```python
from build123d import *

# Parameters (mm, degrees)
EXTRUDE_1_DEPTH          = 60
CUT_EXTRUDE_1_DEPTH      = 40
CUT_EXTRUDE_1_DEPTH_BACK = 29
SKETCH_4_R               = 15.5
SKETCH_5_W               = 5
SKETCH_5_H               = 30
CUT_EXTRUDE_2_DEPTH      = 83.900874001
CUT_EXTRUDE_START        = 25
SKETCH_6_W               = 60
SKETCH_6_H               = 56
CUT_EXTRUDE_3_DEPTH      = 10
CUT_EXTRUDE_START_2      = -15
SKETCH_7_W               = 60
SKETCH_7_H               = 56
CUT_EXTRUDE_4_DEPTH      = 10


with BuildPart() as part:
    # 스케치3 → 보스-돌출1 (new body)
    with BuildSketch(Plane(origin=(0, 0, 0), x_dir=(0, 0, -1), z_dir=(1, 0, 0))):
        Polygon((-25, -51.454396413), (25, -51.454396413), (15, 4.545603587), (-15, 4.545603587), align=None)
    extrude(amount=EXTRUDE_1_DEPTH)

    # 스케치4 → 컷-돌출1 (cut, two sides: drawn at the far end of the back side and taken through both)
    with BuildSketch(Plane.XY.offset(-CUT_EXTRUDE_1_DEPTH_BACK)):
        with Locations(Location((30, -14.954396413, 0), (0, 0, 90))):
            Circle(SKETCH_4_R)
    extrude(amount=CUT_EXTRUDE_1_DEPTH + CUT_EXTRUDE_1_DEPTH_BACK, mode=Mode.SUBTRACT)

    # 스케치5 → 컷-돌출2 (cut, through all)
    with BuildSketch(Plane(origin=(0, 0, 0), x_dir=(0, 0, -1), z_dir=(1, 0, 0))):
        with Locations((0, -51.454396413)):
            Rectangle(SKETCH_5_W, SKETCH_5_H)
    extrude(amount=CUT_EXTRUDE_2_DEPTH, mode=Mode.SUBTRACT)

    # 스케치6 → 컷-돌출3 (cut)
    with BuildSketch(Plane.XY.offset(CUT_EXTRUDE_START)):
        with Locations((30, -23.454396413)):
            Rectangle(SKETCH_6_W, SKETCH_6_H)
    extrude(amount=-CUT_EXTRUDE_3_DEPTH, mode=Mode.SUBTRACT)

    # 스케치7 → 컷-돌출4 (cut)
    with BuildSketch(Plane.XY.offset(CUT_EXTRUDE_START_2)):
        with Locations((30, -23.454396413)):
            Rectangle(SKETCH_7_W, SKETCH_7_H)
    extrude(amount=-CUT_EXTRUDE_4_DEPTH, mode=Mode.SUBTRACT)


solid = part.part
```
CAD build for the part. Positions are in the model's coordinates, mm. A direction names the side the tool comes from. Coordinates: 2 decimals unless noted, no trailing zeros. Order: outer loops, then holes, each group sorted by start corner. A loop starts at its lowest first (then second) coordinate and runs counter-clockwise, first axis right, second up.
(1) Saw through at B-B, the plane x = 30. Write the cut outline in (y, z), and give its area (3 significant figures).
Solution:
outline: (-51.45, -15) - (-30.45, -15) - (-30.45, 15) - (-51.45, 15) - (-51.45, 2.5) - (-36.45, 2.5) - (-36.45, -2.5) - (-51.45, -2.5) - close; (0.55, -15) - (4.55, -15) - (4.55, 15) - (0.55, 15) - close
area: 675 mm2
(2) Drill centre lines: L1, parallel to Z at x = 50, y = -47.5; L2, parallel to X at y = -6.5, z = -7; L3, parallel to Y at x = 17, z = 5.75. Where is each one in solid material? Low to high.
Solution:
L1: z = -15 to -2.5, 2.5 to 15
L2: x = 0 to 17.01, 42.99 to 60
L3: y = -51.45 to -23.4, -6.51 to 4.55
(3) Which spindle directions (+Z, -Z, +X, -X, +Y, -Y) get a long thin tool onto all of the face, cutting with end or side? Do faces 1 (the face through (30, -36.454, 0)), 2 (the face through (30, -51.454, 9)). Say none if no direction does.
Solution:
face 1: +X, -X, -Y
face 2: +Z, -Z, +X, -X, -Y
(4) Saw through at A-A, the plane y = -45. Write the cut outline in (x, z), and give its area (3 significant figures).
Solution:
outline: (0, -15) - (60, -15) - (60, -2.5) - (0, -2.5) - close; (0, 2.5) - (60, 2.5) - (60, 15) - (0, 15) - close
area: 1,500 mm2
(5) Mould opens along Y. For faces 3 (the face through (30, -51.454, -9)), 4 (the face through (35.937, -0.636, -0.21)), 5 (the face through (30, -44, 2.5)) say: released by +Y, released by -Y, zero draft, split by the parting line, or undercut.
Solution:
face 3: released by -Y
face 4: undercut
face 5: zero draft
(6) Saw through at C-C, the plane z = 0.5. Write the cut outline in (x, y), and give its area (3 significant figures).
Solution:
outline: (0, -36.45) - (60, -36.45) - (60, 4.55) - (0, 4.55) - close; hole circle Ø31 at (30, -14.95)
area: 1,710 mm2
(7) Pin check, flat tips, straight feed: pin 1 Ø1.5 at (x, z) = (28, 1) entering from -Y; pin 2 Ø10 at (x, y) = (29, -9) entering from -Z. Stop position of each tip, or through.
Solution:
pin 1: stops at y = -36.45
pin 2: passes through
(8) Saw through at D-D, the plane x = 6. Write the cut outline in (y, z).
Solution:
outline: (-51.45, -15) - (4.55, -15) - (4.55, 15) - (-51.45, 15) - (-51.45, 2.5) - (-36.45, 2.5) - (-36.45, -2.5) - (-51.45, -2.5) - close
